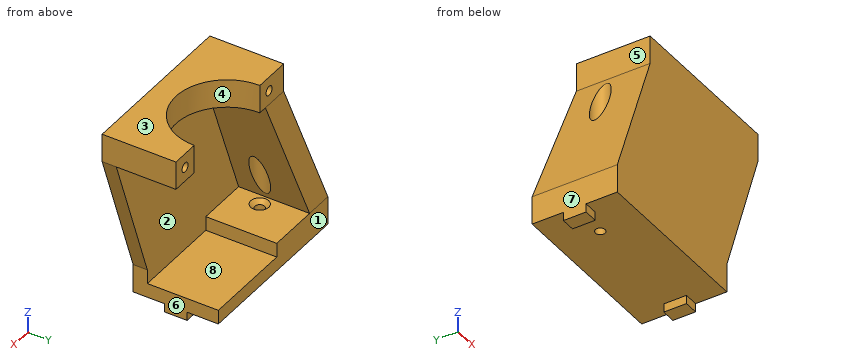
from build123d import *

# Parameters (mm, degrees)
SKETCH_1_W          = 60
SKETCH_1_H          = 30
EXTRUDE_1_DEPTH     = 10
SKETCH_2_W          = 42
SKETCH_2_H          = 42
CUT_EXTRUDE_1_DEPTH = 5
EXTRUDE_2_DEPTH     = 10
CUT_EXTRUDE_2_REACH = 102.96
SKETCH_8_R          = 3.25
SKETCH_9_W          = 5
SKETCH_9_H          = 8
EXTRUDE_3_DEPTH     = 3


# Read off the part's stored shape, not the designer's step: the other step, the other step
with BuildPart() as part:
    # Sketch 1 → Extrude 1 (new body)
    with BuildSketch(Plane.XY):
        with Locations((30, 15)):
            Rectangle(SKETCH_1_W, SKETCH_1_H)
    extrude(amount=EXTRUDE_1_DEPTH)

    # Sketch 2 → Cut-Extrude 1 (cut)
    with BuildSketch(Plane.XY.offset(10)):
        with Locations((49, 26)):
            Rectangle(SKETCH_2_W, SKETCH_2_H)
    extrude(amount=-CUT_EXTRUDE_1_DEPTH, mode=Mode.SUBTRACT)



with BuildPart() as body_2:
    # Sketch 3 → Extrude 2 (new body)
    with BuildSketch(Plane.XY.offset(58)):
        with BuildLine():
            Line((18, 0), (18, 26))
            Line((18, 26), (31, 26))
            ThreePointArc((31, 26), (49, 8), (67, 26))
            Line((67, 26), (77, 26))
            Line((77, 26), (77, 0))
            Line((77, 0), (18, 0))
        make_face()
    extrude(amount=EXTRUDE_2_DEPTH)


with BuildPart() as part_1:
    add(part.part)

    add(body_2.part)  # Loft 1 merges body 2
    # Sketch 5 → Loft 1 section 0
    with BuildSketch(Plane.XY.offset(10)):
        with BuildLine():
            Line((60, 5), (60, 0))
            Line((60, 0), (0, 0))
            Line((0, 0), (0, 30))
            Line((0, 30), (10, 30))
            Line((10, 30), (10, 5))
            Line((10, 5), (60, 5))
        make_face()
    # Sketch 4 → Loft 1 section 1
    with BuildSketch(Plane(origin=(0, 0, 58), x_dir=(-1, 0, 0), z_dir=(0, 0, -1))):
        with BuildLine():
            Line((-18, 26), (-18, 0))
            Line((-18, 0), (-77, 0))
            Line((-77, 0), (-77, 5))
            Line((-77, 5), (-28, 5))
            Line((-28, 5), (-28, 26))
            Line((-28, 26), (-18, 26))
        make_face()
    loft()

    # Other 1 outline → Other 1 (revolve, cut)
    with BuildSketch(Plane(origin=(14, 15, 0), x_dir=(1, 0, 0), z_dir=(0, -1, 0))):
        Polygon((3.15, 10), (0, 10), (0, 0), (1.7, 0), (1.7, 8.55), align=None)
    revolve(axis=Axis((14, 15, 0), (0, 0, 1)), mode=Mode.SUBTRACT)

    # Cut-Extrude 2: up to this plane
    cut_extrude_2_end = Plane(origin=(-3.287671233, 0, 1.232876712), z_dir=(-0.9363291775690445, 0, 0.35112344158839154))
    # Sketch 8 → Cut-Extrude 2 (cut, up to the surface)
    with BuildSketch(Plane.XY.offset(10), mode=Mode.PRIVATE) as cut_extrude_2_sk1:
        with Locations(Location((14, 15, 0), (0, 0, 180))):
            Circle(SKETCH_8_R)
    cut_extrude_2_tool1 = split(extrude(cut_extrude_2_sk1.sketch, amount=CUT_EXTRUDE_2_REACH, mode=Mode.PRIVATE), bisect_by=cut_extrude_2_end, keep=Keep.BOTH, mode=Mode.PRIVATE)
    add(cut_extrude_2_tool1.solids().sort_by_distance((14, 15, 10))[0], mode=Mode.SUBTRACT)

    # Sketch 9 → Extrude 3 (add)
    with BuildSketch(Plane(origin=(0, 0, 0), x_dir=(-1, 0, 0), z_dir=(0, 0, -1))):
        with Locations((-57.5, 15)):
            Rectangle(SKETCH_9_W, SKETCH_9_H)
        with Locations((-2.5, 15)):
            Rectangle(SKETCH_9_W, SKETCH_9_H)
    extrude(amount=EXTRUDE_3_DEPTH)

    # Other 2 outline → Other 2 (revolve, cut)
    with BuildSketch(Plane(origin=(72, 0, 63), x_dir=(1, 0, 0), z_dir=(0, 0, 1))):
        Polygon((0, 15.008579979), (1.65, 16), (1.65, 26), (0, 26), align=None)
    revolve(axis=Axis((72, 0, 63), (0, 1, 0)), mode=Mode.SUBTRACT)

    # Other 2 2 outline → Other 2 2 (revolve, cut)
    with BuildSketch(Plane(origin=(26, 0, 63), x_dir=(1, 0, 0), z_dir=(0, 0, 1))):
        Polygon((0, 15.008579979), (1.65, 16), (1.65, 26), (0, 26), align=None)
    revolve(axis=Axis((26, 0, 63), (0, 1, 0)), mode=Mode.SUBTRACT)


solid = part_1.part
Work out the finished part from the listing and answer in its coordinate system (mm). Face numbers are marked on the shaded views. A direction names the side the tool comes from. Give positions to 0.01 mm unless a question says otherwise; leave off trailing zeros. Answer in a Markdown table with one row per item.
(1) A tool of negligible diameter and unlimited length cuts with its end or side. For the marked faces 4, 5, 6, 7 and 8, from which of +Z, -Z, +X, -X, +Y, -Y can it reach the whole face along a straight path? Write none if from no direction.
Results list:
| item | result |
|---|---|
| face 4 | +Z, +Y |
| face 5 | +Z, -X, +Y, -Y |
| face 6 | -Z, +X, +Y, -Y |
| face 7 | +Z, -Z, -X, +Y, -Y |
| face 8 | +X, +Y |
(2) Consider L1, parallel to Y at x = 45, z = 34.5; L2, parallel to Y at x = 14, z = 4; L3, parallel to X at y = 23.25, z = 63. Determine where each line is inside the solid, lowest interval first. Write a range as [from, to].
Results list:
| item | result |
|---|---|
| L1 | y = [0, 5] |
| L2 | y = [0, 13.3], [16.7, 30] |
| L3 | x = [18, 24.35], [27.65, 31.21], [66.79, 70.35], [73.65, 77] |
(3) Flat-ended cylindrical pins translate along their axes: pin 1 Ø3 at (y, z) = (16, 64) entering from -X; pin 2 Ø6 at (y, z) = (9, 43) entering from +X; pin 3 Ø4 at (x, z) = (72, 63) entering from +Y. Find the tip coordinate at first contact, or state that the pin passes through.
Results list:
| item | result |
|---|---|
| pin 1 | stops at x = 18 |
| pin 2 | stops at x = 23.5 |
| pin 3 | stops at y = 26 |
(4) For a pull along Z with two mould halves and no side action, classify the marked faces 1, 2 and 3 as pulls with the +Z half, pulls with the -Z half, needs draft (parallel to the pull), parting line crosses it, or undercut.
Results list:
| item | result |
|---|---|
| face 1 | needs draft |
| face 2 | undercut |
| face 3 | pulls with the +Z half |
(5) Section A-A (x = 14) is taken. State how many separate pieces and enclosed holes the cut face has, and give its area (3 significant figures).
Results list:
| item | result |
|---|---|
| separate pieces | 3 |
| enclosed holes | 0 |
| area | 891 mm² |
